```python
from build123d import *

# Parameters (mm, degrees)
F1_DEPTH = 50
F2_R     = 15
F2_R_2   = 10
F3_DEPTH = 15
F2_R_3   = 5
F4_DEPTH = 12
F5_DEPTH = 25


with BuildPart() as f1:
    # F0 (on Front) → F1 (new body)
    with BuildSketch(Plane.XZ):
        Polygon((0, 20), (0, 0), (10, 0), (10, 10.000004), (100, 10.000004), (100, 20), align=None)
    extrude(amount=F1_DEPTH)

    # F2 (on face) → F3 (join)
    with BuildSketch(Plane.XY.offset(20)):
        with Locations((70, -25)):
            Circle(F2_R)
        with Locations((70, -25)):
            Circle(F2_R_2, mode=Mode.SUBTRACT)
    extrude(amount=F3_DEPTH)

    # F2 (on face) → F4 (join)
    with BuildSketch(Plane.XY.offset(20)):
        with Locations((70, -25)):
            Circle(F2_R_2)
        with Locations((70, -25)):
            Circle(F2_R_3, mode=Mode.SUBTRACT)
    extrude(amount=F4_DEPTH)

    # F2 (on face) → F5 (cut)
    with BuildSketch(Plane.XY.offset(20)):
        with Locations((70, -25)):
            Circle(F2_R_3)
        with Locations((30, -35)):
            Circle(F2_R_3)
        with Locations((30, -15)):
            Circle(F2_R_3)
    extrude(amount=-F5_DEPTH, mode=Mode.SUBTRACT)


solid = f1.part
```
Geometry check sheet. Reference: the model listing, model coordinates, mm. A direction names the side the tool comes from. Coordinates: 2 decimals unless noted, no trailing zeros. Order: outer loops, then holes, each group sorted by start corner. A loop starts at its lowest first (then second) coordinate and runs counter-clockwise, first axis right, second up.
Q1. Sectioned sample at C-C on x = 70. Record the cut outline in (y, z), and give its area (3 significant figures).
Reply:
outline: (-50, 10) - (-30, 10) - (-30, 32) - (-35, 32) - (-35, 35) - (-40, 35) - (-40, 20) - (-50, 20) - close; (-20, 10) - (0, 10) - (0, 20) - (-10, 20) - (-10, 35) - (-15, 35) - (-15, 32) - (-20, 32) - close
area: 670 mm2
Q2. Depth check by flat-ended pin: pin 1 Ø8 at (x, y) = (84, -22.5) entering from -Z; pin 2 Ø5 at (x, y) = (18, -12) entering from +Z; pin 3 Ø10 at (x, y) = (68.5, -23) entering from +Z. Enter the tip coordinate at first touch or a pass-through.
Reply:
pin 1: stops at z = 10
pin 2: stops at z = 20
pin 3: stops at z = 32
Q3. Draft check along Y on faces 4 (the face through (54, -25, 10)), 5 (the face through (58, -34, 27)), 6 (the face through (60, -25, 33)), 7 (the face through (49, -50, 15)). Enter one of: released by +Y, released by -Y, zero draft, split by the parting line, or undercut.
Reply:
face 4: zero draft
face 5: split by the parting line
face 6: undercut
face 7: released by -Y
Q4. Sectioned sample at A-A on y = -25. Record the cut outline in (x, z), and give its area (3 significant figures).
Reply:
outline: (0, 0) - (10, 0) - (10, 10) - (65, 10) - (65, 32) - (60, 32) - (60, 35) - (55, 35) - (55, 20) - (0, 20) - close; (75, 10) - (100, 10) - (100, 20) - (85, 20) - (85, 35) - (80, 35) - (80, 32) - (75, 32) - close
area: 1,270 mm2
Q5. Thickness scan on probe 1 along Y at (x, z) = (30, 15); probe 2 along Z at (x, y) = (10.5, -7.5); probe 3 along X at (y, z) = (-13.5, 14). Record the ranges inside material, lowest first.
Reply:
probe 1: y = -50 to -40, -30 to -20, -10 to 0
probe 2: z = 10 to 20
probe 3: x = 0 to 25.23, 34.77 to 100
Q6. Sectioned sample at B-B on z = 12.5. Record the cut outline in (x, y), and give its area (3 significant figures).
Reply:
outline: (0, -50) - (100, -50) - (100, 0) - (0, 0) - close; hole circle Ø10 at (30, -35); hole circle Ø10 at (30, -15); hole circle Ø10 at (70, -25)
area: 4,760 mm2
Q7. Sectioned sample at D-D on y = -17. Record the cut outline in (x, z), and give its area (3 significant figures).
Reply:
outline: (0, 0) - (10, 0) - (10, 10) - (25.42, 10) - (25.42, 20) - (0, 20) - close; (34.58, 10) - (100, 10) - (100, 20) - (82.69, 20) - (82.69, 35) - (76, 35) - (76, 32) - (64, 32) - (64, 35) - (57.31, 35) - (57.31, 20) - (34.58, 20) - close
area: 1,350 mm2
Q8. Tool access check on faces 1 (the face through (65, -27, 32)), 2 (the face through (5, -25, 0)), 3 (the face through (10, -25, 5)). Record the directions out of +Z, -Z, +X, -X, +Y, -Y that give a thin tool (end or side, any length) a straight path to the whole face; none if there is none.
Reply:
face 1: +Z
face 2: -Z, +X, -X, +Y, -Y
face 3: -Z, +X, +Y, -Y
